Verification items for the finished model (mm, model axes). Face numbers are marked on the shaded views. A direction names the side the tool comes from. Round coordinates to 2 decimals unless told otherwise and drop trailing zeros. Order: outer loops, then holes, each group sorted by start corner. A loop starts at its lowest first (then second) coordinate and runs counter-clockwise, first axis right, second up. Notation, with made-up numbers: (72.5, 31.25) -> (109.5, 31.25) arc R9 cw to (109.5, 36.25) -> close; hole circle Ø7 at (83.5, 68). An arc over 180 degrees is marked (long way). Put each result on its own line as item: value.
```python
from build123d import *

# Parameters (mm, degrees)
F0_W     = 69.2
F0_H     = 44.2
F1_DEPTH = 20
F2_R     = 3
F3_T     = -1.6
F4_R     = 2
F5_DEPTH = 3
F6_W     = 15.5
F6_H     = 10.5
F7_DEPTH = 1.6
F8_W     = 10
F8_H     = 4
F9_DEPTH = 1.6


with BuildPart() as f1:
    # F0 (on Top) → F1 (new body)
    with BuildSketch(Plane.XY):
        Rectangle(F0_W, F0_H)
    extrude(amount=F1_DEPTH)

    # F2
    f2_edges = [f1.edges().sort_by_distance(p)[0] for p in [
        (34.6, -22.1, 10),
        (34.6, 22.1, 10),
        (-34.6, 22.1, 10),
        (-34.6, -22.1, 10),
    ]]
    fillet(f2_edges, radius=F2_R)

    # F3
    f3_openings = [f1.faces().sort_by_distance(p)[0] for p in [
        (0, 0, 20),
    ]]
    offset(amount=F3_T, openings=f3_openings)

    # F4 (on face) → F5 (join)
    with BuildSketch(Plane.XY.offset(1.6)):
        with Locations((-30, 18)):
            Circle(F4_R)
        with Locations((30, 18)):
            Circle(F4_R)
        with Locations((30, -18)):
            Circle(F4_R)
        with Locations((-30, -18)):
            Circle(F4_R)
    extrude(amount=F5_DEPTH)

    # F6 (on face) → F7 (cut, through all)
    with BuildSketch(Plane.YZ.offset(34.6)):
        with Locations((-1.95, 11.25)):
            Rectangle(F6_W, F6_H)
    extrude(amount=-F7_DEPTH, mode=Mode.SUBTRACT)

    # F8 (on face) → F9 (cut, through all)
    with BuildSketch(Plane(origin=(-34.6, 0, 0), x_dir=(0, -1, 0), z_dir=(-1, 0, 0))):
        with Locations((-7.9, 12.1)):
            Rectangle(F8_W, F8_H)
    extrude(amount=-F9_DEPTH, mode=Mode.SUBTRACT)


solid = f1.part
```
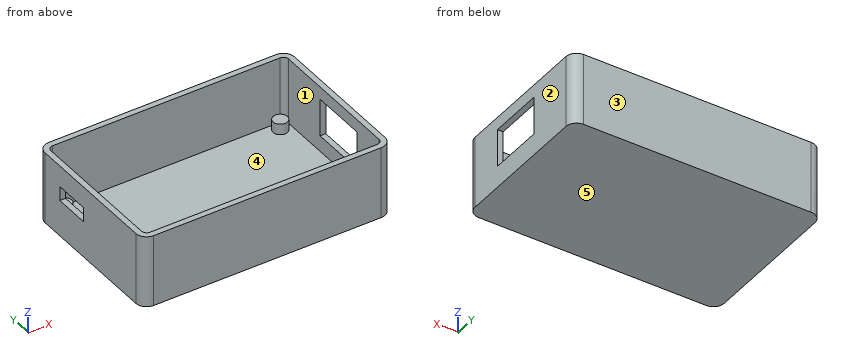
Item 1: Release check for a two-part mould opening along Z. For the marked faces 3, 4 and 5 record: pulls with the +Z half, pulls with the -Z half, needs draft (parallel to the pull), parting line crosses it, or undercut.
Geometry check:
face 3: needs draft
face 4: pulls with the +Z half
face 5: pulls with the -Z half
Item 2: Depth check by flat-ended pin: pin 1 Ø2 at (x, y) = (29, -18.5) entering from +Z; pin 2 Ø12 at (x, y) = (11, 1.5) entering from +Z; pin 3 Ø0.8 at (x, z) = (-33.5, 12.5) entering from +Y; pin 4 Ø4 at (y, z) = (9.5, 13.5) entering from -X. Enter the tip coordinate at first touch or a pass-through.
Geometry check:
pin 1: z = 4.6
pin 2: z = 1.6
pin 3: y = 21.7
pin 4: x = -34.6
Item 3: Material ranges on line 1 along X through (y, z) = (3.5, 18.5); line 2 along Y through (x, z) = (7, 15.5); line 3 along X through (y, z) = (17.5, 3.75), recorded low to high.
Geometry check:
line 1: -34.6 to -33, 33 to 34.6
line 2: -22.1 to -20.5, 20.5 to 22.1
line 3: -34.6 to -33, -31.94 to -28.06, 28.06 to 31.94, 33 to 34.6
Item 4: Sectioned sample at D-D, the plane x = 24.5. Record the boundary of the cut face in (y, z), then the cut area to 3 significant figures.
Geometry check:
outline: (-22.1, 0) -> (22.1, 0) -> (22.1, 20) -> (20.5, 20) -> (20.5, 1.6) -> (-20.5, 1.6) -> (-20.5, 20) -> (-22.1, 20) -> close
area: 130 mm2
Item 5: Tool access check on the marked faces 1 and 2. Record the directions out of +Z, -Z, +X, -X, +Y, -Y that give a thin tool (end or side, any length) a straight path to the whole face; none if there is none.
Geometry check:
face 1: +Z
face 2: +Z, -Z, +X, +Y, -Y
Item 6: Sectioned sample at C-C, the plane z = 18. Record the boundary of the cut face in (x, y).
Geometry check:
outline: (-34.6, -19.1) arc R3 ccw to (-31.6, -22.1) -> (31.6, -22.1) arc R3 ccw to (34.6, -19.1) -> (34.6, 19.1) arc R3 ccw to (31.6, 22.1) -> (-31.6, 22.1) arc R3 ccw to (-34.6, 19.1) -> close; hole (-33, -19.1) arc R1.4 ccw to (-31.6, -20.5) -> (31.6, -20.5) arc R1.4 ccw to (33, -19.1) -> (33, 19.1) arc R1.4 ccw to (31.6, 20.5) -> (-31.6, 20.5) arc R1.4 ccw to (-33, 19.1) -> close
Item 7: Sectioned sample at A-A, the plane y = -2. Record the boundary of the cut face in (x, z).
Geometry check:
outline: (-34.6, 0) -> (34.6, 0) -> (34.6, 6) -> (33, 6) -> (33, 1.6) -> (-33, 1.6) -> (-33, 20) -> (-34.6, 20) -> close; (33, 16.5) -> (34.6, 16.5) -> (34.6, 20) -> (33, 20) -> close
Item 8: Sectioned sample at B-B, the plane z = 11. Record the boundary of the cut face in (x, y).
Geometry check:
outline: (-34.6, -19.1) arc R3 ccw to (-31.6, -22.1) -> (31.6, -22.1) arc R3 ccw to (34.6, -19.1) -> (34.6, -9.7) -> (33, -9.7) -> (33, -19.1) arc R1.4 cw to (31.6, -20.5) -> (-31.6, -20.5) arc R1.4 cw to (-33, -19.1) -> (-33, 2.9) -> (-34.6, 2.9) -> close; (-34.6, 12.9) -> (-33, 12.9) -> (-33, 19.1) arc R1.4 cw to (-31.6, 20.5) -> (31.6, 20.5) arc R1.4 cw to (33, 19.1) -> (33, 5.8) -> (34.6, 5.8) -> (34.6, 19.1) arc R3 ccw to (31.6, 22.1) -> (-31.6, 22.1) arc R3 ccw to (-34.6, 19.1) -> close
